Autodesk Inventor part; units mm, degrees
ref_plane "YZ Plane" through (0, 0, 0) normal (1, 0, 0) x (0, 1, 0)
ref_plane "XZ Plane" through (0, 0, 0) normal (0, 1, 0) x (-1, 0, 0)
ref_plane "XY Plane" through (0, 0, 0) normal (0, 0, 1) x (1, 0, 0)
sketch "Sketch1" plane through (0, 0, 0) normal (0, 0, 1) x (1, 0, 0)
  circle A0 centre (0, 0) radius 28.575
  circle A1 centre (0, 0) radius 23.8125
  circle A2 centre (0, 0) radius 12.7
  point P0 (20.6222, -11.9063)
  point P1 (20.6222, 11.9062)
  point P2 (0, 23.8125)
  point P3 (-20.6222, 11.9063)
  point P4 (-20.6222, -11.9062)
  point P5 (0, -23.8125)
  dimension "d1" = 47.625
  dimension "d0" = 57.15
  dimension "d4" = 360
  dimension "d6" = 25.4
extrude "Extrusion1" add sketch "Sketch1" along normal blind 6.35 contours A0 | A1
hole "Hole1" at (20.6222, -11.9063, 0) at (20.6222, 11.9062, 0) at (0, 23.8125, 0) at (-20.6222, 11.9063, 0) at (-20.6222, -11.9062, 0) at (0, -23.8125, 0) direction (0, 0, 1) diameter 5.08 end through all
properties part number "lower box hub"
The model under review builds one solid part; all positions refer to its coordinate system, in mm. Round coordinates to 2 decimals unless told otherwise and drop trailing zeros. Loops run counter-clockwise (first coordinate to the right, second up) from the corner with the lowest first, then second, coordinate; pieces in that order, holes last. Notation, with made-up numbers: M 55.25,-22.75 L 111.25,-22.75 A28 ccw 111.25,4.25 Z; hole C 8.5,-12.5 d9. An arc over 180 degrees is marked long. Answer as a JSON object with one key per item and string values.
Item 1: For line 1 along Y through (x, z) = (0, 2.5) (1 decimal); line 2 along Y through (x, z) = (21.5, 1.5); line 3 along X through (y, z) = (14, 1.5), list the stretches that pass through material, from the lowest coordinate up.
Check sheet entries:
{"line 1": "-28.6 to -26.4, -21.3 to -12.7, 12.7 to 21.3, 26.4 to 28.6", "line 2": "-18.82 to -14.29, -9.52 to 9.52, 14.29 to 18.82", "line 3": "-24.91 to -22.06, -19.18 to 19.18, 22.06 to 24.91"}
Item 2: We need section C-C, the plane x = 0. State how many separate pieces and enclosed holes the cut face has, and give its area (3 significant figures).
Check sheet entries:
{"separate pieces": "4", "enclosed holes": "0", "area": "137 mm2"}
Item 3: The part is to be moulded in two halves that separate along Y. For faces 1 (the face through (-28.547, -1.256, 3.131)), 2 (the face through (-22.339, -13.778, 3.219)), 3 (the face through (12, -6, 0)), 4 (the face through (-2.75, 12.4, 3.13)), say which applies: +Y half, -Y half, draft (parallel to the pull), parting line (faces both ways), or undercut.
Check sheet entries:
{"face 1": "parting line", "face 2": "undercut", "face 3": "draft", "face 4": "undercut"}
Item 4: We need section B-B, the plane x = -12. State the section outline as (y, z) points.
Check sheet entries:
{"outline": "M -25.93,0 L -4.16,0 L -4.16,6.35 L -25.93,6.35 Z; M 4.16,0 L 25.93,0 L 25.93,6.35 L 4.16,6.35 Z"}
Item 5: Clearance check with flat-ended pins moving along their axes: P1, Ø3, axis at x = -17.5, z = 3.5, coming from the +Y side; P2, Ø1.5, axis at y = 7.5, z = 2, coming from the -X side; P3, Ø2, axis at y = -10.5, z = 3, coming from the +X side; P4, Ø4.5, axis at x = 0, y = 23.81, coming from the -Z side. State where each tip first meets the part, or that it passes through.
Check sheet entries:
{"P1": "y = 23.68", "P2": "x = -27.77", "P3": "x = 26.95", "P4": "through"}
Item 6: We need section D-D, the plane y = -11. State the section outline as (x, z) points (3 decimals), and give its area (3 significant figures).
Check sheet entries:
{"outline": "M -26.373,0 L -22.995,0 L -22.995,6.35 L -26.373,6.35 Z; M -18.249,0 L -6.347,0 L -6.347,6.35 L -18.249,6.35 Z; M 6.347,0 L 18.249,0 L 18.249,6.35 L 6.347,6.35 Z; M 22.995,0 L 26.373,0 L 26.373,6.35 L 22.995,6.35 Z", "area": "194 mm2"}
Item 7: We need section A-A, the plane y = 0. State the section outline as (x, z) points (3 decimals).
Check sheet entries:
{"outline": "M -28.575,0 L -12.7,0 L -12.7,6.35 L -28.575,6.35 Z; M 12.7,0 L 28.575,0 L 28.575,6.35 L 12.7,6.35 Z"}
